from build123d import *

# Parameters (mm, degrees)
SKETCH_1_W          = 15
SKETCH_1_H          = 15
SKETCH_1_W_2        = 13
SKETCH_1_H_2        = 13
EXTRUDE_1_DEPTH     = 230
SKETCH_2_R          = 1.45
CUT_EXTRUDE_1_DEPTH = 231.610602532


with BuildPart() as part:
    # 草图1 → 凸台-拉伸1 (new body)
    with BuildSketch(Plane(origin=(0, 0, 0), x_dir=(0, 0, -1), z_dir=(1, 0, 0))):
        Rectangle(SKETCH_1_W, SKETCH_1_H)
        Rectangle(SKETCH_1_W_2, SKETCH_1_H_2, mode=Mode.SUBTRACT)
    extrude(amount=EXTRUDE_1_DEPTH)

    # 草图2 → 切除-拉伸1 (cut, through all)
    with BuildSketch(Plane.XZ.offset(7.5)):
        with Locations(Location((215, 0, 0), (0, 0, 270))):
            Circle(SKETCH_2_R)
        with Locations(Location((225, 0, 0), (0, 0, 270))):
            Circle(SKETCH_2_R)
        with Locations(Location((164.69848481, 0, 0), (0, 0, 270))):
            Circle(SKETCH_2_R)
        with Locations(Location((139.69848481, 0, 0), (0, 0, 270))):
            Circle(SKETCH_2_R)
        with Locations(Location((5, 0, 0), (0, 0, 270))):
            Circle(SKETCH_2_R)
        with Locations(Location((15, 0, 0), (0, 0, 270))):
            Circle(SKETCH_2_R)
        with Locations(Location((115, 0, 0), (0, 0, 270))):
            Circle(SKETCH_2_R)
        with Locations(Location((90.3, 0, 0), (0, 0, 270))):
            Circle(SKETCH_2_R)
        with Locations(Location((34, 0, 0), (0, 0, 270))):
            Circle(SKETCH_2_R)
        with Locations(Location((44, 0, 0), (0, 0, 270))):
            Circle(SKETCH_2_R)
        with Locations(Location((54, 0, 0), (0, 0, 270))):
            Circle(SKETCH_2_R)
    extrude(amount=-CUT_EXTRUDE_1_DEPTH, mode=Mode.SUBTRACT)


solid = part.part
Design review of the part built by this model. Coordinates are the model's own, in mm. A direction names the side the tool comes from. Coordinates: 2 decimals unless noted, no trailing zeros. Order: outer loops, then holes, each group sorted by start corner. A loop starts at its lowest first (then second) coordinate and runs counter-clockwise, first axis right, second up. Notation, with made-up numbers: M -27,9.25 L 18,9.25 A15 ccw 18,23.25 Z; hole C 23,80.25 d7. An arc over 180 degrees is marked long. Use a Markdown table: item, result.
(1) Add section B-B (z = 3.5). Give the boundary of the cut face in (x, y), then the cut area to 3 significant figures.
Worked answers:
| item | result |
|---|---|
| outline | M 0,-7.5 L 230,-7.5 L 230,-6.5 L 0,-6.5 Z; M 0,6.5 L 230,6.5 L 230,7.5 L 0,7.5 Z |
| area | 460 mm2 |
(2) Wall thickness on probe 1 along Z at (x, y) = (115, -6.9); probe 2 along Z at (x, y) = (34.5, -0.5): over which ranges is each line inside the solid? List them lowest first.
Worked answers:
| item | result |
|---|---|
| probe 1 | z = -7.5 to -1.45, 1.45 to 7.5 |
| probe 2 | z = -7.5 to -6.5, 6.5 to 7.5 |
(3) Add section A-A (x = 60). Give the boundary of the cut face in (y, z), then the cut area to 3 significant figures.
Worked answers:
| item | result |
|---|---|
| outline | M -7.5,-7.5 L 7.5,-7.5 L 7.5,7.5 L -7.5,7.5 Z; hole M -6.5,-6.5 L 6.5,-6.5 L 6.5,6.5 L -6.5,6.5 Z |
| area | 56.0 mm2 |
(4) For faces 4 (the flat face through (113, 0, 7.5)), 5 (the flat face through (113, 6.5, 0)), list the 3-axis set-ups (+Z, -Z, +X, -X, +Y, -Y) from which the entire face can be reached by the end or side of a thin tool; tool diameter is ignored.
Worked answers:
| item | result |
|---|---|
| face 4 | +Z, +X, -X, +Y, -Y |
| face 5 | +X, -X |
(5) Draft analysis for pull direction Z (two halves, no side actions). For faces 1 (the flat face through (113, 0, -7.5)), 2 (the flat face through (113, 0, 6.5)), 3 (the flat face through (113, 7.5, 0)), state which applies: released by +Z, released by -Z, zero draft, split by the parting line, or undercut.
Worked answers:
| item | result |
|---|---|
| face 1 | released by -Z |
| face 2 | undercut |
| face 3 | zero draft |
